Print and shaded views of the part. All mm, measured from the part's lowest x, y and z. A direction names the side the tool comes from. Coordinates: 2 decimals unless noted, no trailing zeros. Write each loop counter-clockwise with the first axis right and the second up, starting at its lowest first coordinate (ties: lowest second). Pieces come first, ordered by that corner, then holes. Notation, with made-up numbers: (73, 69.25) -> (106, 69.25) arc R11 cw to (106, 78.25) -> close; hole circle Ø11 at (-6, -25). An arc over 180 degrees is marked (long way). Write item = value, one per line.
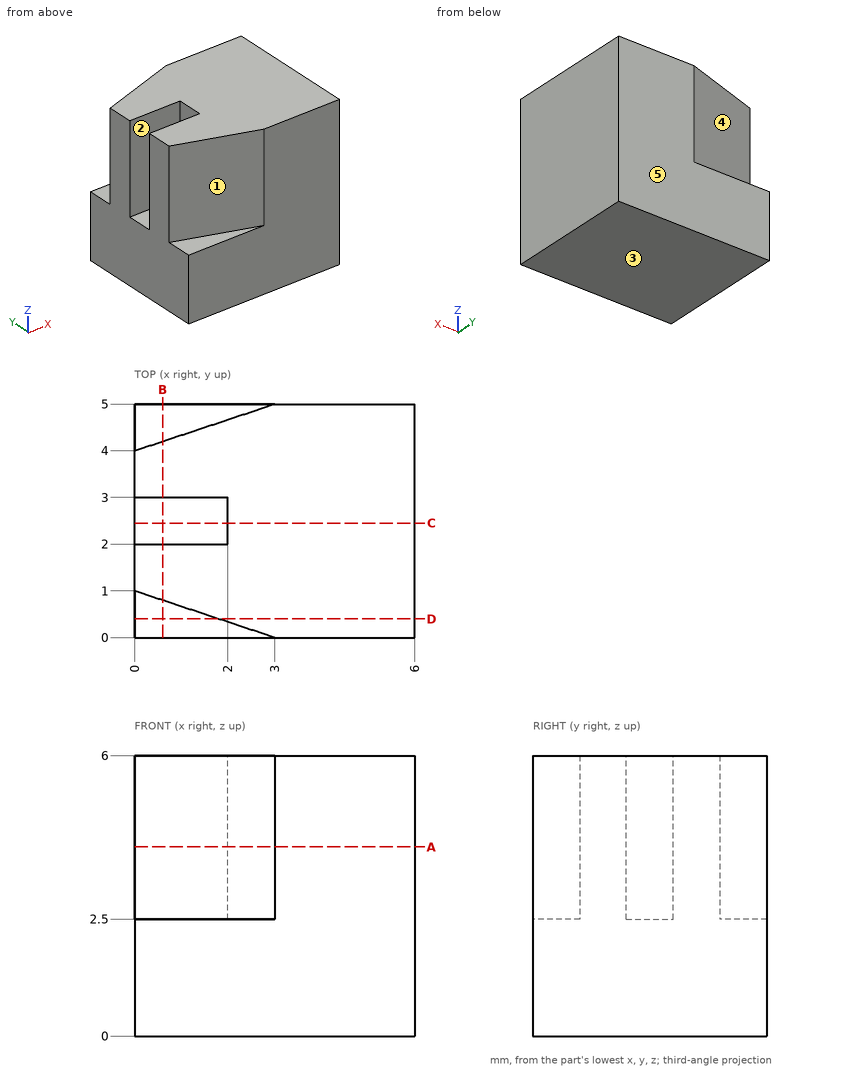
Q1. Which spindle directions (+Z, -Z, +X, -X, +Y, -Y) get a long thin tool onto all of the face, cutting with end or side? Do the marked faces 4 and 5. Say none if no direction does.
Model answer:
face_4 = +Z, -X, +Y
face_5 = +Z, -Z, +X, -X, +Y
Q2. Pin check, flat tips, straight feed: pin 1 (1.5 mm diameter, centred on x = 2, z = 4.5, fed in from -Y); pin 2 (1 mm diameter, centred on x = 1, z = 3.5, fed in from -Y); pin 3 (1 mm diameter, centred on x = 1, z = 4, fed in from +Y). Stop position of each tip, or through.
Model answer:
pin_1 = 0.08
pin_2 = 0.5
pin_3 = 4.5
Q3. Probe line 1 (Y direction, x = 0.6, z = 5.6); line 2 (X direction, y = 2.95, z = 3.15); line 3 (Y direction, x = 1.55, z = 3.7). List the from-to ranges inside material, lowest first. Write a range as from..to.
Model answer:
line_1 = 0.8..2, 3..4.2
line_2 = 2..6
line_3 = 0.48..2, 3..4.52
Q4. Saw through at B-B on x = 0.6. Give the cut face in (y, z), and give its area (3 significant figures).
Model answer:
outline = (0, 0) -> (5, 0) -> (5, 2.5) -> (4.2, 2.5) -> (4.2, 6) -> (3, 6) -> (3, 2.5) -> (2, 2.5) -> (2, 6) -> (0.8, 6) -> (0.8, 2.5) -> (0, 2.5) -> close
area = 20.9 mm²
Q5. Saw through at A-A on z = 4.05. Give the cut face in (x, y).
Model answer:
outline = (0, 1) -> (3, 0) -> (6, 0) -> (6, 5) -> (3, 5) -> (0, 4) -> (0, 3) -> (2, 3) -> (2, 2) -> (0, 2) -> close
Q6. Saw through at D-D on y = 0.4. Give the cut face in (x, z).
Model answer:
outline = (0, 0) -> (6, 0) -> (6, 6) -> (1.8, 6) -> (1.8, 2.5) -> (0, 2.5) -> close
Q7. Saw through at C-C on y = 2.45. Give the cut face in (x, z), and give its area (3 significant figures).
Model answer:
outline = (0, 0) -> (6, 0) -> (6, 6) -> (2, 6) -> (2, 2.5) -> (0, 2.5) -> close
area = 29.0 mm²
Q8. Mould opens along Y. For the marked faces 1, 2 and 3 say: released by +Y, released by -Y, zero draft, split by the parting line, or undercut.
Model answer:
face_1 = released by -Y
face_2 = undercut
face_3 = zero draft
